Autodesk Inventor part; units mm, degrees
ref_plane "YZ Plane" through (0, 0, 0) normal (1, 0, 0) x (0, 1, 0)
ref_plane "XZ Plane" through (0, 0, 0) normal (0, 1, 0) x (-1, 0, 0)
ref_plane "XY Plane" through (0, 0, 0) normal (0, 0, 1) x (1, 0, 0)
sketch "スケッチ1" plane through (0, 0, 0) normal (0, 0, 1) x (1, 0, 0)
  circle A0 centre (0, 0) radius 40.5
  circle A1 centre (0, 440) radius 40.5
  line L0 (-40.5, 0) -> (-40.5, 440)
  line L1 (40.5, 440) -> (40.5, 0)
  dimension "d0" = 81
  dimension "d1" = 81
  dimension "d2" = 440
extrude "プレート1" add sketch "スケッチ1" along normal blind 2
sketch "スケッチ4" plane through (0, 0, 0) normal (0, 0, -1) x (-1, 0, 0)
  circle A0 centre (0, 0) radius 28
  dimension "d28" = 56
extrude "押し出し1" cut sketch "スケッチ4" against normal blind 10
sketch "スケッチ5" plane through (0, 0, 0) normal (0, 0, -1) x (-1, 0, 0)
  circle A0 centre (0, 0) radius 32
  point P0 (0, 32)
  point P1 (-27.7128, 16)
  point P2 (-27.7128, -16)
  point P3 (0, -32)
  point P4 (27.7128, -16)
  point P5 (27.7128, 16)
  dimension "d31" = 64
  dimension "d34" = 360
hole "穴3" at (0, 32, 0) at (27.7128, 16, 0) at (27.7128, -16, 0) at (0, -32, 0) at (-27.7128, -16, 0) at (-27.7128, 16, 0) direction (0, 0, 1) diameter 4.3 end through all
sketch "スケッチ6" plane through (0, 0, 2) normal (0, 0, 1) x (1, 0, 0)
  arc A0 (40.5, 440) -> (-40.5, 440) centre (0, 440) ccw
  circle A1 centre (0, 440) radius 32.55
  point P0 (0, 0)
  dimension "d43" = 65.1
extrude "押し出し2" cut sketch "スケッチ6" against normal blind 10
sketch "スケッチ9" plane through (0, 0, 2) normal (0, 0, 1) x (1, 0, 0)
  arc A0 (40.5, 440) -> (-40.5, 440) centre (0, 440) ccw
  circle A1 centre (0, 440) radius 36.5
  point P0 (0, 0)
  point P1 (0, 476.5)
  point P2 (-31.6099, 458.25)
  point P3 (-31.6099, 421.75)
  point P4 (0, 403.5)
  point P5 (31.6099, 421.75)
  point P6 (31.6099, 458.25)
  dimension "d58" = 73
  dimension "d61" = 360
hole "穴5" at (0, 476.5, 2) at (-31.6099, 458.25, 2) at (-31.6099, 421.75, 2) at (0, 403.5, 2) at (31.6099, 421.75, 2) at (31.6099, 458.25, 2) direction (0, 0, -1) diameter 3.2 end through all
sketch "スケッチ16" plane through (0, 0, 2) normal (0, 0, 1) x (1, 0, 0)
  circle A0 centre (0, 355.2097) radius 4
  arc A1 (40.5, 440) -> (-40.5, 440) centre (0, 440) ccw
  circle A2 centre (0, 440) radius 25
  line L0 (-23.4923, 431.4495) -> (4.1883, 355.3977)
  line L1 (0, 603.9) -> (0, -147.9)
  point P0 (0, 0)
  dimension "d154" = 50
  dimension "d135" = 8
  dimension "d136" = 0
  dimension "d137" = 160
hole "穴11" at (0, 355.2097, 2) direction (0, 0, -1) diameter 4.5 end through all
sketch "スケッチ17" plane through (0, 0, 2) normal (0, 0, 1) x (1, 0, 0)
  circle A0 centre (0, 0) radius 44
  point P0 (-4, 72)
  dimension "d145" = 88
  dimension "d177" = 72
  dimension "d178" = 4
hole "穴12" at (-4, 72, 2) direction (0, 0, -1) diameter 4.3 end through all
sketch "スケッチ18" plane through (0, 0, 0) normal (0, 0, -1) x (-1, 0, 0)
  line L0 (-9, 41) -> (9, 41)
  line L1 (9, 41) -> (9, 56)
  line L2 (9, 56) -> (-9, 56)
  line L3 (-9, 56) -> (-9, 41)
  line L4 (-9, 41) -> (9, 56) construction
  line L5 (9, 41) -> (-9, 56) construction
  arc A0 (40.5, 440) -> (-40.5, 440) centre (0, 440) ccw
  point P0 (0, 0)
  point P1 (0, 48.5)
  point P2 (0, 48.5)
  dimension "d157" = 18
  dimension "d158" = 15
  dimension "d183" = 41
extrude "押し出し4" cut sketch "スケッチ18" against normal blind 10
fillet "コーナーR2" radius 2 4 edges at (-9, 56, 1) (9, 56, 1) (9, 41, 1) (-9, 41, 1)
sketch "スケッチ19" plane through (0, 0, 2) normal (0, 0, 1) x (1, 0, 0)
  line L0 (21, 72) -> (-4, 72) construction
  line L1 (21, 69.85) -> (-4, 69.85)
  line L2 (-4, 74.15) -> (21, 74.15)
  arc A0 (21, 69.85) -> (21, 74.15) centre (21, 72) ccw
  arc A1 (-4, 74.15) -> (-4, 69.85) centre (-4, 72) ccw
  circle A2 centre (-4, 72) radius 2.15
  point P0 (0, 0)
  point P1 (8.5, 72)
  dimension "d182" = 21
extrude "押し出し5" cut sketch "スケッチ19" against normal blind 10
sketch "スケッチ20" plane through (0, 0, 0) normal (0, 0, -1) x (-1, 0, 0)
  point P0 (0, 0)
  point P1 (0, 220)
  dimension "d167" = 220
hole "穴13" at (0, 220, 0) direction (0, 0, 1) diameter 4.3 end through all
equation "\"d41\" = Thickness"
equation "\"d68\" = Thickness"
equation "\"d143\" = Thickness"
equation "\"d152\" = Thickness"
equation "\"d173\" = Thickness"
equation "\"d3\" = Thickness"
equation "\"BendRadius\" = Thickness"
equation "\"BendReliefWidth\" = Thickness"
equation "\"BendReliefDepth\" = 0.5 * Thickness"
equation "\"CornerReliefSize\" = 4 * Thickness"
equation "\"MinimumRemnant\" = 2 * Thickness"
equation "\"TransitionRadius\" = BendRadius"
equation "\"JacobiRadiusSize\" = Thickness"
equation "\"GapSize\" = Thickness"
properties part number "link2-plate2" material "CFRP"
For this review, take the finished solid that the model builds, in its own axes (mm). Give positions to 0.01 mm unless a question says otherwise; leave off trailing zeros. Loops run counter-clockwise (first coordinate to the right, second up) from the corner with the lowest first, then second, coordinate; pieces in that order, holes last.
Item 1: Take a section at B-B, the plane z = 0.8. Give the number of separate pieces and of enclosed holes in the cut face, and give its area (3 significant figures).
Item 2: Take a section at A-A, the plane y = 413. State the section outline as (x, z) points, and give its area (3 significant figures).
Item 3: Draft analysis for pull direction Y (two halves, no side actions). For faces 1 (the cylindrical face through (0.89, -40.49, 0.99)), 2 (the cylindrical face through (-7.056, 408.224, 1.014)), 3 (the cylindrical face through (-0.89, 480.49, 0.99)), 4 (the flat face through (-1, 224, 0)), state which applies: +Y half, -Y half, draft (parallel to the pull), parting line (faces both ways), or undercut.
Item 4: For line 1 along Y through (x, z) = (-7.5, 0.25); line 2 along Y through (x, z) = (-19, 0.15); line 3 along X through (y, z) = (420.5, 0.5), list the stretches that pass through material, from the lowest coordinate up.
Item 5: Insertion check: pin 1 (1 mm diameter, centred on x = -18.5, z = 0.5, fed in from -Y). The pin has a flat end and moves straight along its axis. Give the tip position at first contact, or say it passes through.
Calculated:
1. separate pieces: 1
1. enclosed holes: 18
1. area: 34,400 mm2
2. outline: (-40.5, 0) - (-18.18, 0) - (-18.18, 2) - (-40.5, 2) - close; (18.18, 0) - (40.5, 0) - (40.5, 2) - (18.18, 2) - close
2. area: 89.3 mm2
3. face 1: -Y half
3. face 2: undercut
3. face 3: +Y half
3. face 4: draft
4. line 1: y = -39.8 to -26.98, 26.98 to 41.06, 55.94 to 408.33, 471.67 to 479.8
4. line 2: y = -35.77 to -20.57, 20.57 to 413.57, 466.43 to 475.77
4. line 3: x = -40.5 to -32.61, -30.61 to -26.06, 26.06 to 30.61, 32.61 to 40.5
5. pin 1: stops at y = -36.28
